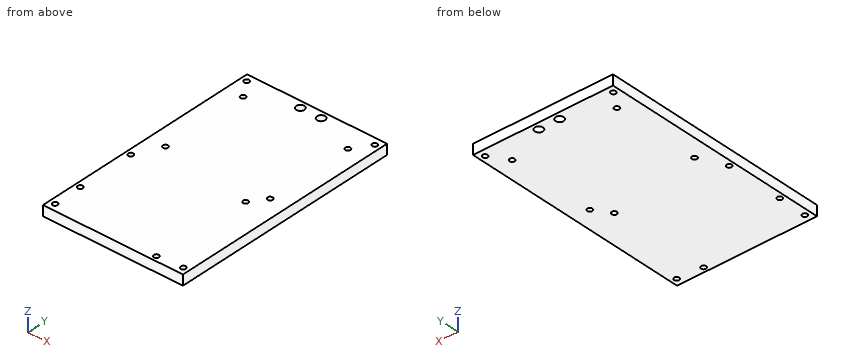
```python
from build123d import *

# Parameters (mm, degrees)
SKETCH1_W                        = 68.600000001
SKETCH1_H                        = 113.65
BRACKETBASE_DEPTH                = 5
ARDUINOMOUNTINGHOLES_DEPTH       = 22
ARDUINOMOUNTINGHOLES_DEPTH_BACK  = 120.777809299
ARDUINOMOUNTINGHOLESSKETCH_R     = 1.25
F_9VBATTERYMOUNTINGHOLESSKETCH_R = 1.25
F_9VBATTERYMOUNTINGHOLES_DEPTH   = 20
LEGBRACKETMOUNTINGHOLESSKETCH_R  = 2
LEGBRACKETMOUNTINGHOLES_DEPTH    = 13
BACKSIDEMOUNTINGHOLESSKETCH_R    = 1.25
BACKSIDEMOUNTINGHOLES_DEPTH      = 24


with BuildPart() as part:
    # Sketch1 → bracketBase (new body)
    with BuildSketch(Plane.XY):
        with Locations((34.3, 41.235000001)):
            Rectangle(SKETCH1_W, SKETCH1_H)
    extrude(amount=BRACKETBASE_DEPTH)

    # arduinoMountingHolesSketch → arduinoMountingHoles (cut, two sides: drawn at the far end of the back side and taken through both)
    with BuildSketch(Plane.XY.offset(-ARDUINOMOUNTINGHOLES_DEPTH_BACK)):
        with Locations((2.54, 2.280000001)):
            Circle(ARDUINOMOUNTINGHOLESSKETCH_R)
        with Locations((2.54, 30.450000001)):
            Circle(ARDUINOMOUNTINGHOLESSKETCH_R)
        with Locations((54.600000001, 35.270000001)):
            Circle(ARDUINOMOUNTINGHOLESSKETCH_R)
        with Locations((53.350000001, -13.049999999)):
            Circle(ARDUINOMOUNTINGHOLESSKETCH_R)
    extrude(amount=ARDUINOMOUNTINGHOLES_DEPTH + ARDUINOMOUNTINGHOLES_DEPTH_BACK, mode=Mode.SUBTRACT)

    # 9VbatteryMountingHolesSketch → 9VbatteryMountingHoles (cut)
    with BuildSketch(Plane.XY):
        with Locations((8.625000001, 86.060000001)):
            Circle(F_9VBATTERYMOUNTINGHOLESSKETCH_R)
        with Locations(Location((59.975000001, 86.060000001, 0), (0, 0, 180))):
            Circle(F_9VBATTERYMOUNTINGHOLESSKETCH_R)
        with Locations(Location((8.625000001, 42.810000001, 0), (0, 0, 180))):
            Circle(F_9VBATTERYMOUNTINGHOLESSKETCH_R)
        with Locations((59.975000001, 42.810000001)):
            Circle(F_9VBATTERYMOUNTINGHOLESSKETCH_R)
    extrude(amount=F_9VBATTERYMOUNTINGHOLES_DEPTH, mode=Mode.SUBTRACT)

    # legBracketMountingHolesSketch → legBracketMountingHoles (cut)
    with BuildSketch(Plane.XY):
        with Locations((29.202551646, 94.560000001)):
            Circle(LEGBRACKETMOUNTINGHOLESSKETCH_R)
        with Locations(Location((39.397448356, 94.560000001, 0), (0, 0, 180))):
            Circle(LEGBRACKETMOUNTINGHOLESSKETCH_R)
    extrude(amount=LEGBRACKETMOUNTINGHOLES_DEPTH, mode=Mode.SUBTRACT)

    # backsideMountingHolesSketch → backsideMountingHoles (cut)
    with BuildSketch(Plane.XY):
        with Locations((2.875000001, 94.560000001)):
            Circle(BACKSIDEMOUNTINGHOLESSKETCH_R)
        with Locations(Location((65.725000001, 94.560000001, 0), (0, 0, 180))):
            Circle(BACKSIDEMOUNTINGHOLESSKETCH_R)
        with Locations((65.725000001, -12.089999999)):
            Circle(BACKSIDEMOUNTINGHOLESSKETCH_R)
        with Locations(Location((2.875000001, -12.089999999, 0), (0, 0, 180))):
            Circle(BACKSIDEMOUNTINGHOLESSKETCH_R)
    extrude(amount=BACKSIDEMOUNTINGHOLES_DEPTH, mode=Mode.SUBTRACT)


solid = part.part
```
Work out the finished part from the listing and answer in its coordinate system (mm). Give positions to 0.01 mm unless a question says otherwise; leave off trailing zeros. Loops run counter-clockwise (first coordinate to the right, second up) from the corner with the lowest first, then second, coordinate; pieces in that order, holes last. Notation, with made-up numbers: (56, 5.25) -> (109, 5.25) arc R22 ccw to (109, 34.25) -> close; hole circle Ø8 at (-24, 69.25). An arc over 180 degrees is marked (long way). Put each result on its own line as item: value. Start each with the question number.
Item 1: Each of these flat-tipped pins is pushed along its axis until it touches: P1, Ø2.5, axis at x = 29.2, y = 94.56, coming from the +Z side; P2, Ø3, axis at x = 2.875, y = 94.56, coming from the +Z side. Where does it stop, or does it pass through?
Item 2: The part is cut by section A-A (y = 86.06). Give the vertices of the cut face in (x, z) (3 decimals).
Item 3: Find the intervals of material crossed by L1, parallel to Y at x = 60, z = 3.45; L2, parallel to X at y = 85, z = 3.8; L3, parallel to X at y = 29.5, z = 0.35, in increasing order. Write a range as [from, to].
Item 4: The part is cut by section B-B (y = 2.28). Give the vertices of the cut face in (x, z).
Answers below:
1. P1: through
1. P2: z = 5
2. outline: (0, 0) -> (7.375, 0) -> (7.375, 5) -> (0, 5) -> close; (9.875, 0) -> (58.725, 0) -> (58.725, 5) -> (9.875, 5) -> close; (61.225, 0) -> (68.6, 0) -> (68.6, 5) -> (61.225, 5) -> close
3. L1: [-15.59, 41.56], [44.06, 84.81], [87.31, 98.06]
3. L2: [0, 7.96], [9.29, 59.31], [60.64, 68.6]
3. L3: [0, 1.73], [3.35, 68.6]
4. outline: (0, 0) -> (1.29, 0) -> (1.29, 5) -> (0, 5) -> close; (3.79, 0) -> (68.6, 0) -> (68.6, 5) -> (3.79, 5) -> close
